The figure shows three views and two pictorial views of one solid part (mm, origin at its lowest corner). Answer the questions. Round coordinates to 2 decimals unless told otherwise and drop trailing zeros. Order: outer loops, then holes, each group sorted by start corner. A loop starts at its lowest first (then second) coordinate and runs counter-clockwise, first axis right, second up. Notation, with made-up numbers: (-18.75, 57) -> (19.25, 57) arc R21 ccw to (19.25, 72) -> close; hole circle Ø9 at (-14, 42). An arc over 180 degrees is marked (long way). Return JSON: item names as keys, results as strings. Group by question number.
(1) The part is cut by section C-C (x = 80). Determine the outline of the cut face in (y, z), plus the area to 3 significant figures.
(2) The part is cut by section B-B (z = 7). Determine the outline of the cut face in (x, y), plus the area to 3 significant figures.
(3) Consider line 1 (Y direction, x = 150.5, z = 3); line 2 (Y direction, x = 450, z = 9); line 3 (X direction, y = 55.5, z = 10.75). Determine where each line is inside the solid, lowest interval first. Write a range as [from, to].
(4) The part is cut by section A-A (y = 70). Determine the outline of the cut face in (x, z), plus the area to 3 significant figures.
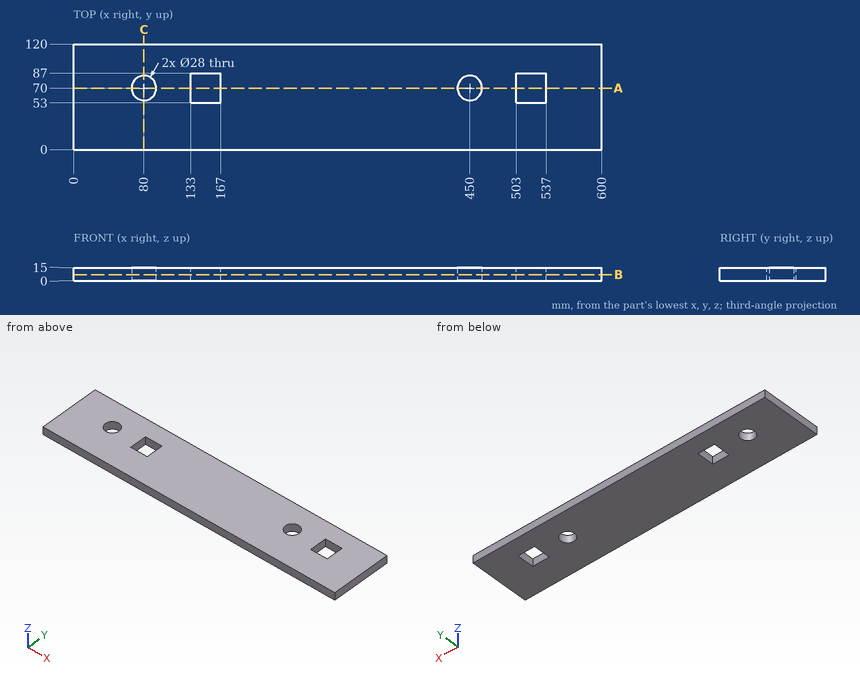
Answer below:
{
 "1": {"outline": "(0, 0) -> (56, 0) -> (56, 15) -> (0, 15) -> close; (84, 0) -> (120, 0) -> (120, 15) -> (84, 15) -> close", "area": "1,380 mm²"},
 "2": {"outline": "(0, 0) -> (600, 0) -> (600, 120) -> (0, 120) -> close; hole circle Ø28 at (80, 70); hole (133, 53) -> (167, 53) -> (167, 87) -> (133, 87) -> close; hole circle Ø28 at (450, 70); hole (503, 53) -> (537, 53) -> (537, 87) -> (503, 87) -> close", "area": "68,500 mm²"},
 "3": {"line 1": "y = [0, 53], [87, 120]", "line 2": "y = [0, 56], [84, 120]", "line 3": "x = [0, 133], [167, 503], [537, 600]"},
 "4": {"outline": "(0, 0) -> (66, 0) -> (66, 15) -> (0, 15) -> close; (94, 0) -> (133, 0) -> (133, 15) -> (94, 15) -> close; (167, 0) -> (436, 0) -> (436, 15) -> (167, 15) -> close; (464, 0) -> (503, 0) -> (503, 15) -> (464, 15) -> close; (537, 0) -> (600, 0) -> (600, 15) -> (537, 15) -> close", "area": "7,140 mm²"}
}
